Autodesk Inventor part; units mm, degrees
ref_plane "YZ Plane" through (0, 0, 0) normal (1, 0, 0) x (0, 1, 0)
ref_plane "XZ Plane" through (0, 0, 0) normal (0, 1, 0) x (-1, 0, 0)
ref_plane "XY Plane" through (0, 0, 0) normal (0, 0, 1) x (1, 0, 0)
sketch "Sketch1" plane through (0, 0, 0) normal (0, 0, 1) x (1, 0, 0)
  line L0 (0, 50.8) -> (12.7, 50.8)
  line L1 (12.7, 50.8) -> (12.7, 0)
  line L2 (12.7, 0) -> (0, 0)
  line L3 (0, 0) -> (0, 50.8)
  dimension "d0" = 12.7
  dimension "d1" = 50.8
extrude "Extrusion1" add sketch "Sketch1" along normal blind 1.778
sketch "Sketch2" plane through (0, 0, 1.778) normal (0, 0, 1) x (1, 0, 0)
  line L0 (12.7, 0) -> (0, 0)
  circle A0 centre (6.35, 9.525) radius 1.9844
  dimension "d4" = 3.9688
  dimension "d5" = 9.525
extrude "Extrusion2" cut sketch "Sketch2" against normal through all
pattern_linear "Rectangular Pattern1" count 2 spacing 31.75 along (0, 1, 0) of "Extrusion2"
properties part number "SM-M05" material "Steel, Mild"
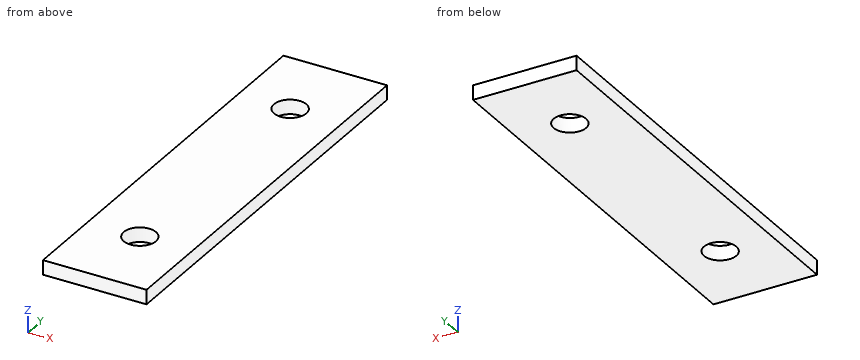
Check sheet for the modelled part. Datum: model origin and axes. Units: mm. Coordinates: 2 decimals unless noted, no trailing zeros. Order: outer loops, then holes, each group sorted by start corner. A loop starts at its lowest first (then second) coordinate and runs counter-clockwise, first axis right, second up. Notation, with made-up numbers: (-8.5, -27.75) -> (46.5, -27.75) arc R13 cw to (46.5, -16.75) -> close; hole circle Ø7 at (-39, 8). An arc over 180 degrees is marked (long way). Write item = value, one per line. Start each with the question number.
1) Cross-section at C-C (z = 0.4). Enter the section's corners in (x, y) (3 decimals), then the cut area to 3 significant figures.
2) Cross-section at B-B (y = 8). Enter the section's corners in (x, z), then the cut area to 3 significant figures.
3) Cross-section at A-A (x = 6.35). Enter the section's corners in (y, z).
4) Go/stop test with a flat-tipped pin: P1, Ø2.5, axis at x = 6.35, y = 41.275, coming from the -Z side. Record where the tip stops, or that it passes through.
5) Material ranges on L1, parallel to Y at x = 6.35, z = 1.4; L2, parallel to Y at x = 5.5, z = 1.6; L3, parallel to X at y = 39.5, z = 1.35, recorded low to high.
Ans:
q1.outline = (0, 0) -> (12.7, 0) -> (12.7, 50.8) -> (0, 50.8) -> close; hole circle Ø3.969 at (6.35, 9.525); hole circle Ø3.969 at (6.35, 41.275)
q1.area = 620 mm²
q2.outline = (0, 0) -> (5.08, 0) -> (5.08, 1.78) -> (0, 1.78) -> close; (7.62, 0) -> (12.7, 0) -> (12.7, 1.78) -> (7.62, 1.78) -> close
q2.area = 18.1 mm²
q3.outline = (0, 0) -> (7.54, 0) -> (7.54, 1.78) -> (0, 1.78) -> close; (11.51, 0) -> (39.29, 0) -> (39.29, 1.78) -> (11.51, 1.78) -> close; (43.26, 0) -> (50.8, 0) -> (50.8, 1.78) -> (43.26, 1.78) -> close
q4.P1 = through
q5.L1 = 0 to 7.54, 11.51 to 39.29, 43.26 to 50.8
q5.L2 = 0 to 7.73, 11.32 to 39.48, 43.07 to 50.8
q5.L3 = 0 to 5.46, 7.24 to 12.7
